Model file for the job. Use its own axes, mm. Face numbers are marked on the shaded views. Give positions to 0.01 mm unless a question says otherwise; leave off trailing zeros. Write each loop counter-clockwise with the first axis right and the second up, starting at its lowest first coordinate (ties: lowest second). Pieces come first, ordered by that corner, then holes. Notation, with made-up numbers: (59.25, 38) - (68.25, 38) arc R17 cw to (68.25, 70) - close; hole circle Ø2 at (-38, -19.5). An arc over 180 degrees is marked (long way). Use CSV: the item, a comma, the result in double quotes.
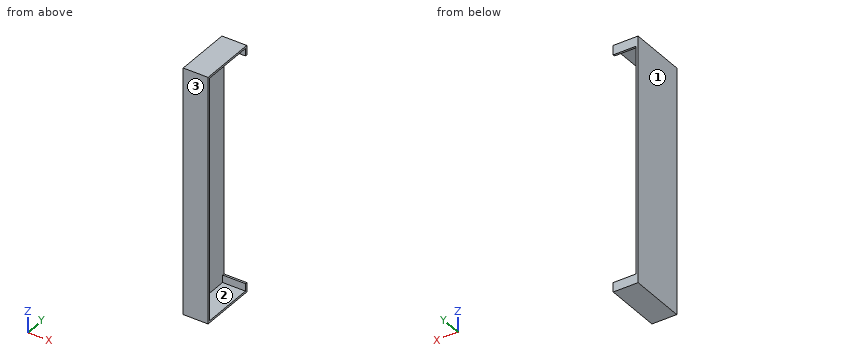
from build123d import *

# Parameters (mm, degrees)
SALIENTE_EXTRUIR1_DEPTH      = 248
SALIENTE_EXTRUIR1_DEPTH_BACK = 248
CROQUIS2_W                   = 50
CROQUIS2_H                   = 115
SALIENTE_EXTRUIR2_DEPTH      = 4
CROQUIS5_W                   = 46
CROQUIS5_H                   = 15
SALIENTE_EXTRUIR5_DEPTH      = 4


with BuildPart() as part:
    # Croquis1 → Saliente-Extruir1 (new body, two sides)
    with BuildSketch(Plane.XY) as saliente_extruir1_sk:
        Polygon((0, 0), (0, 115), (4, 115), (4, 4), (50, 4), (50, 0), align=None)
    extrude(amount=SALIENTE_EXTRUIR1_DEPTH)
    extrude(saliente_extruir1_sk.sketch, amount=-SALIENTE_EXTRUIR1_DEPTH_BACK)

    # Croquis2 → Saliente-Extruir2 (add)
    with BuildSketch(Plane.XY.offset(248)):
        with Locations((25, 57.5)):
            Rectangle(CROQUIS2_W, CROQUIS2_H)
    saliente_extruir2 = extrude(amount=-SALIENTE_EXTRUIR2_DEPTH)

    # Simetr_a1: Saliente-Extruir2 across plane
    add(saliente_extruir2.mirror(Plane.XY))

    # Croquis5 → Saliente-Extruir5 (add)
    with BuildSketch(Plane(origin=(0, 115, 0), x_dir=(1, 0, 0), z_dir=(0, 1, 0))):
        with Locations((27, -236.5)):
            Rectangle(CROQUIS5_W, CROQUIS5_H)
    saliente_extruir5 = extrude(amount=-SALIENTE_EXTRUIR5_DEPTH)

    # Simetr_a2: Saliente-Extruir5 across plane
    add(saliente_extruir5.mirror(Plane.XY))


solid = part.part
(1) Saw through at A-A, the plane x = 26. List the corners of the cut face in (y, z).
Checked values:
outline,"(0, -248) - (115, -248) - (115, -229) - (111, -229) - (111, -244) - (4, -244) - (4, 244) - (111, 244) - (111, 229) - (115, 229) - (115, 248) - (0, 248) - close"
(2) Saw through at C-C, the plane z = 104. List the corners of the cut face in (x, y).
Checked values:
outline,"(0, 0) - (50, 0) - (50, 4) - (4, 4) - (4, 115) - (0, 115) - close"
(3) Saw through at B-B, the plane y = 73. List the corners of the cut face in (x, z), then the cut area to 3 significant figures.
Checked values:
outline,"(0, -248) - (50, -248) - (50, -244) - (4, -244) - (4, 244) - (50, 244) - (50, 248) - (0, 248) - close"
area,"2,350 mm^2"
(4) Pull direction Y, two halves, no side cores. Call the marked faces 1, 2 and 3: released by +Y, released by -Y, zero draft, split by the parting line, or undercut.
Checked values:
face 1,"zero draft"
face 2,"undercut"
face 3,"released by -Y"
(5) Flat gauge pins, fed straight in: P1, Ø5, axis at y = 100.5, z = 5.5, coming from the +X side; P2, Ø2, axis at x = 42, z = -134, coming from the +Y side. Where does each tip first touch, or does it go through?
Checked values:
P1,"stops at x = 4"
P2,"stops at y = 4"
(6) Wall check: probe 1 along Z at (x, y) = (17, 61); probe 2 along Y at (x, z) = (7.5, 173.5). Give the ranges that are in metal, low to high. Write a range as [from, to].
Checked values:
probe 1,"z = [-248, -244], [244, 248]"
probe 2,"y = [0, 4]"
